from build123d import *

# Parameters (mm, degrees)
F0_R           = 11.90625
F1_DEPTH       = 25.4
F2_D           = 7.1374
F2_CBORE_D     = 11.1125
F2_CBORE_DEPTH = 6.35
F3_SIZE        = 0.254


with BuildPart() as f1:
    # F0 (on Top) → F1 (new body)
    with BuildSketch(Plane.XY):
        Circle(F0_R)
    extrude(amount=F1_DEPTH)

    # F2 (through all)
    with Locations(Plane(origin=(0, 0, 0), x_dir=(1, 0, 0), z_dir=(0, 0, -1))):
        with Locations((0, 0)):
            CounterBoreHole(F2_D / 2, F2_CBORE_D / 2, F2_CBORE_DEPTH)

    # F3
    f3_edges = [f1.edges().sort_by_distance(p)[0] for p in [
        (-11.90625, 0, 25.4),
        (-11.90625, 0, 0),
        (-5.55625, 0, 0),
        (-3.5687, 0, 25.4),
    ]]
    chamfer(f3_edges, length=F3_SIZE)


solid = f1.part
Geometry: final body of the model. Coordinates: model frame, mm. A direction names the side the tool comes from. Coordinates: 2 decimals unless noted, no trailing zeros. Order: outer loops, then holes, each group sorted by start corner. A loop starts at its lowest first (then second) coordinate and runs counter-clockwise, first axis right, second up.
(1) Draft query along X for faces 1 (the face through (0, 4, 6.35)), 2 (the face through (-9.45, -7.24, 12.53)), 3 (the face through (-2.8, 5.3, 0)). Return one class per face: pulls with the +X half, pulls with the -X half, needs draft (parallel to the pull), parting line crosses it, or undercut.
(2) First-contact query: pin 1 (6 mm diameter, centred on x = -7.5, z = 22.5, fed in from -Y); pin 2 (5.5 mm diameter, centred on x = -2, y = -1, fed in from -Z); pin 3 (4 mm diameter, centred on y = 4.5, z = 15, fed in from +X). Flat tips, straight axial feed; report the tip coordinate or a pass-through.
(3) Section query C-C (z = 17.25). Return the cut outline in (x, y), plus the area to 3 significant figures.
(4) Material intervals for probe 1 along Y at (x, z) = (0, 4.25); probe 2 along Y at (x, z) = (0, 19.5); probe 3 along Z at (x, y) = (-3.75, -1), sorted ascending.
(5) Section query A-A (x = 0). Return the cut outline in (y, z), plus the area to 3 significant figures.
(6) Access query for faces 4 (the face through (5.3, -1.67, 3.26)), 5 (the face through (-3, 3, 25.4)). Directions: +Z, -Z, +X, -X, +Y, -Y. A direction counts if a zero-diameter tool reaches every point of the face in a straight line with its end or side. Return the directions, or none.
Solution:
1. face 1: undercut
1. face 2: parting line crosses it
1. face 3: needs draft
2. pin 1: stops at y = -11.02
2. pin 2: stops at z = 6.35
2. pin 3: stops at x = 11.64
3. outline: circle Ø23.81 at (0, 0); hole circle Ø7.14 at (0, 0)
3. area: 405 mm2
4. probe 1: y = -11.91 to -5.56, 5.56 to 11.91
4. probe 2: y = -11.91 to -3.57, 3.57 to 11.91
4. probe 3: z = 6.35 to 25.4
5. outline: (-11.91, 0.25) - (-11.65, 0) - (-5.81, 0) - (-5.56, 0.25) - (-5.56, 6.35) - (-3.57, 6.35) - (-3.57, 25.15) - (-3.82, 25.4) - (-11.65, 25.4) - (-11.91, 25.15) - close; (3.57, 6.35) - (5.56, 6.35) - (5.56, 0.25) - (5.81, 0) - (11.65, 0) - (11.91, 0.25) - (11.91, 25.15) - (11.65, 25.4) - (3.82, 25.4) - (3.57, 25.15) - close
5. area: 398 mm2
6. face 4: -Z
6. face 5: +Z, +X, -X, +Y, -Y
